Verification items for the finished model (mm, model axes). A direction names the side the tool comes from. Give positions to 0.01 mm unless a question says otherwise; leave off trailing zeros. Loops run counter-clockwise (first coordinate to the right, second up) from the corner with the lowest first, then second, coordinate; pieces in that order, holes last. Notation, with made-up numbers: (-14.75, 73) - (1.25, 73) arc R31 ccw to (1.25, 103) - close; hole circle Ø7 at (10, -11). An arc over 180 degrees is marked (long way). One line per item, written item: value. Start each with the question number.
1. Sectioned sample at D-D (x = -12). Record the cut outline in (y, z) (1 decimal).
2. Sectioned sample at A-A (z = 0). Record the cut outline in (x, y) (3 decimals), plus the area to 3 significant figures.
3. Scan lines: L1, parallel to X at y = -12.5, z = 0 (3 decimals); L2, parallel to Y at x = 11, z = 9.5; L3, parallel to Z at x = 8, y = 21. Record each from-to range of solid material in increasing order. Write a range as [from, to].
4. Mould release check, pull along Y, two halves, no side actions. Record for faces 1 (the cylindrical face through (-0.19, 22.69, 21.46)), 2 (the flat face through (10, -5.556, 0)), 3 (the cylindrical face through (15.15, 13.32, 21.46)): pulls with the +Y half, pulls with the -Y half, needs draft (parallel to the pull), parting line crosses it, or undercut.
5. Access from +Z, -Z, +X, -X, +Y, -Y to the whole of each face (thin tool, end or side, straight path). Record for faces 4 (the cylindrical face through (15.11, 13.32, -21.5)), 5 (the flat face through (0, -25, -7.938)), 6 (the flat face through (10, 5.556, 0)), 7 (the flat face through (0, -23.416, 15)).
6. Gauge pin test, flat ends, axial feed: pin 1 (5.5 mm diameter, centred on y = 0, z = -2.5, fed in from +X); pin 2 (11.5 mm diameter, centred on x = -4.76, z = 0, fed in from -Y); pin 3 (7 mm diameter, centred on x = 3.5, z = -16, fed in from -Y); pin 4 (0.7 mm diameter, centred on x = 1.5, y = -24.5, fed in from -Z). Record the tip position at first contact, or that the pin passes through.
7. Sectioned sample at B-B (x = -2). Record the cut outline in (y, z) (1 decimal).
8. Sectioned sample at C-C (y = -15). Record the cut outline in (x, z) (1 decimal), plus the area to 3 significant figures.
from build123d import *

# Parameters (mm, degrees)
BOSS_EXTRUDE1_DEPTH     = 22.225
SKETCH4_W               = 15.875
SKETCH4_H               = 2.38125
BOSS_EXTRUDE2_DEPTH     = 31.75
SKETCH2_R               = 6.33095
CUT_EXTRUDE1_DEPTH      = 1
CUT_EXTRUDE1_DEPTH_BACK = 50.2125
CUT_EXTRUDE2_REACH      = 51.212
SKETCH3_R               = 3.96875
FILLET1_R               = 2.54


with BuildPart() as part:
    # Sketch1 → Boss-Extrude1 (new body, symmetric)
    with BuildSketch(Plane.XY):
        Polygon((15.875, 23.415625), (-15.875, 23.415625), (-15.875, -23.415625), (15.875, -23.415625), (15.875, -5.55625), (3.96875, -5.55625), (3.96875, 5.55625), (15.875, 5.55625), align=None)
    extrude(amount=BOSS_EXTRUDE1_DEPTH, both=True)

    # Sketch4 → Boss-Extrude2 (add, through all)
    with BuildSketch(Plane(origin=(15.875, 0, 0), x_dir=(0, 0, -1), z_dir=(1, 0, 0))):
        with Locations((0, -24.60625)):
            Rectangle(SKETCH4_W, SKETCH4_H)
    extrude(amount=-BOSS_EXTRUDE2_DEPTH)

    # Sketch2 → Cut-Extrude1 (cut, two sides)
    with BuildSketch(Plane(origin=(0, 23.415625, 0), x_dir=(1, 0, 0), z_dir=(0, 1, 0))) as cut_extrude1_sk:
        with Locations((-4.7625, 0)):
            Circle(SKETCH2_R)
    extrude(amount=CUT_EXTRUDE1_DEPTH, mode=Mode.SUBTRACT)
    extrude(cut_extrude1_sk.sketch, amount=-CUT_EXTRUDE1_DEPTH_BACK, mode=Mode.SUBTRACT)

    # Sketch3 → Cut-Extrude2 (cut, up to next)
    with BuildSketch(Plane(origin=(0, 23.415625, 0), x_dir=(1, 0, 0), z_dir=(0, 1, 0)), mode=Mode.PRIVATE) as cut_extrude2_sk1:
        with Locations((8.73125, 14.816666667)):
            Circle(SKETCH3_R)
    cut_extrude2_tool1 = extrude(cut_extrude2_sk1.sketch, amount=-CUT_EXTRUDE2_REACH, mode=Mode.PRIVATE) & part.part
    add(cut_extrude2_tool1.solids().sort_by_distance((8.73125, 23.415625, -14.816667))[0], mode=Mode.SUBTRACT)
    # Sketch3 → Cut-Extrude2 (cut, up to next)
    with BuildSketch(Plane(origin=(0, 23.415625, 0), x_dir=(1, 0, 0), z_dir=(0, 1, 0)), mode=Mode.PRIVATE) as cut_extrude2_sk2:
        with Locations((8.73125, -14.816666667)):
            Circle(SKETCH3_R)
    cut_extrude2_tool2 = extrude(cut_extrude2_sk2.sketch, amount=-CUT_EXTRUDE2_REACH, mode=Mode.PRIVATE) & part.part
    add(cut_extrude2_tool2.solids().sort_by_distance((8.73125, 23.415625, 14.816667))[0], mode=Mode.SUBTRACT)

    # Fillet1
    fillet1_edges = [part.edges().sort_by_distance(p)[0] for p in [
        (15.875, -14.4859375, 22.225),
        (-15.875, 0, -22.225),
        (-15.875, 23.415625, 0),
        (15.875, 23.415625, 0),
        (15.875, 14.4859375, 22.225),
        (0, 23.415625, 22.225),
        (-15.875, 0, 22.225),
        (0, 23.415625, -22.225),
        (15.875, 14.4859375, -22.225),
        (15.875, -14.4859375, -22.225),
    ]]
    fillet(fillet1_edges, radius=FILLET1_R)


solid = part.part
Results are:
1. outline: (-25.8, -7.9) - (-23.4, -7.9) - (-23.4, -22.2) - (20.9, -22.2) arc R2.5 ccw to (23.4, -19.7) - (23.4, 19.7) arc R2.5 ccw to (20.9, 22.2) - (-23.4, 22.2) - (-23.4, 7.9) - (-25.8, 7.9) - close
2. outline: (-15.875, -25.797) - (-11.093, -25.797) - (-11.093, 23.416) - (-13.335, 23.416) arc R2.54 ccw to (-15.875, 20.876) - close; (1.568, -25.797) - (15.875, -25.797) - (15.875, -5.556) - (3.969, -5.556) - (3.969, 5.556) - (15.875, 5.556) - (15.875, 20.876) arc R2.54 ccw to (13.335, 23.416) - (1.568, 23.416) - close
2. area: 804 mm^2
3. L1: x = [-15.875, -11.093], [1.568, 15.875]
3. L2: y = [-23.42, -5.56], [5.56, 23.42]
3. L3: z = [-22.22, -18.72], [-10.92, 10.92], [18.72, 22.22]
4. face 1: pulls with the +Y half
4. face 2: undercut
4. face 3: needs draft
5. face 4: -Z, +X, +Y, -Y
5. face 5: -Z, +X, -X, -Y
5. face 6: +Z, -Z, +X
5. face 7: +Z, +X, -X, -Y
6. pin 1: stops at x = 3.97
6. pin 2: passes through
6. pin 3: stops at y = -23.42
6. pin 4: stops at z = -7.94
7. outline: (-25.8, -7.9) - (-23.4, -7.9) - (-23.4, -22.2) - (20.9, -22.2) arc R2.5 ccw to (23.4, -19.7) - (23.4, -5.7) - (-25.8, -5.7) - close; (-25.8, 5.7) - (23.4, 5.7) - (23.4, 19.7) arc R2.5 ccw to (20.9, 22.2) - (-23.4, 22.2) - (-23.4, 7.9) - (-25.8, 7.9) - close
8. outline: (-15.9, -19.7) arc R2.5 ccw to (-13.3, -22.2) - (13.3, -22.2) arc R2.5 ccw to (15.9, -19.7) - (15.9, 19.7) arc R2.5 ccw to (13.3, 22.2) - (-13.3, 22.2) arc R2.5 ccw to (-15.9, 19.7) - close; hole circle Ø12.7 at (-4.8, 0)
8. area: 1,280 mm^2
